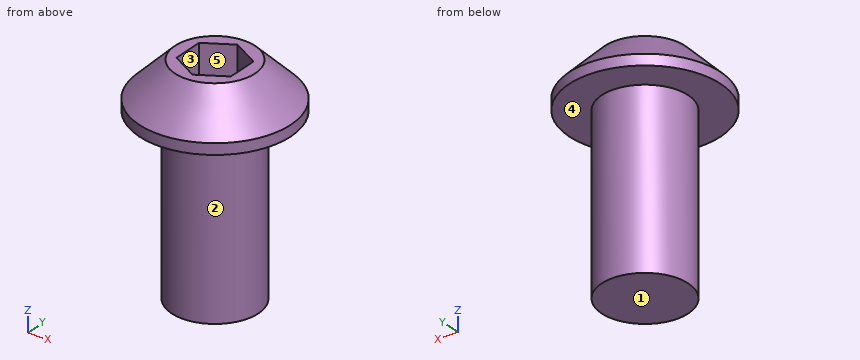
```python
from build123d import *

# Parameters (mm, degrees)
SKETCH1_R           = 7
BASE_EXTRUDE_DEPTH  = 4.3
SKETCH2_R           = 4
BOSS_EXTRUDE1_DEPTH = 16
CUT_EXTRUDE1_DEPTH  = 4.3
CHAMFER1_SIZE       = 3.3


with BuildPart() as part:
    # Sketch1 → Base-Extrude (new body)
    with BuildSketch(Plane.XY):
        Circle(SKETCH1_R)
    extrude(amount=BASE_EXTRUDE_DEPTH)

    # Sketch2 → Boss-Extrude1 (add)
    with BuildSketch(Plane(origin=(0, 0, 0), x_dir=(-1, 0, 0), z_dir=(0, 0, -1))):
        Circle(SKETCH2_R)
    extrude(amount=BOSS_EXTRUDE1_DEPTH)

    # Sketch3 → Cut-Extrude1 (cut)
    with BuildSketch(Plane.XY.offset(4.3)):
        Polygon((0, 2.886751346), (-2.5, 1.443375673), (-2.5, -1.443375673), (0, -2.886751346), (2.5, -1.443375673), (2.5, 1.443375673), align=None)
    extrude(amount=-CUT_EXTRUDE1_DEPTH, mode=Mode.SUBTRACT)

    # Chamfer1
    chamfer1_edges = [part.edges().sort_by_distance(p)[0] for p in [
        (-7, 0, 4.3),
    ]]
    chamfer(chamfer1_edges, length=CHAMFER1_SIZE)


solid = part.part
```
Model file for the job. Use its own axes, mm. Face numbers are marked on the shaded views. A direction names the side the tool comes from. Give positions to 0.01 mm unless a question says otherwise; leave off trailing zeros. Loops run counter-clockwise (first coordinate to the right, second up) from the corner with the lowest first, then second, coordinate; pieces in that order, holes last. Notation, with made-up numbers: (56, -37) - (106, -37) arc R32 ccw to (106, -8) - close; hole circle Ø8 at (39, 53.25). An arc over 180 degrees is marked (long way). One line per item, written item: value. Start each with the question number.
1. Which spindle directions (+Z, -Z, +X, -X, +Y, -Y) get a long thin tool onto all of the face, cutting with end or side? Do the marked faces 4 and 5. Say none if no direction does.
2. Probe L1, parallel to Z at x = 2, y = -1.25; L2, parallel to Y at x = 0, z = -7; L3, parallel to X at y = -2.5, z = 1.25. List the from-to ranges inside material, lowest first. Write a range as from..to.
3. Slice it at B-B (z = -2.5). List the corners of the cut face in (x, y), plus the area to 3 significant figures.
4. Pin check, flat tips, straight feed: pin 1 (3 mm diameter, centred on y = 1, z = -8, fed in from -X); pin 2 (1 mm diameter, centred on y = 5, z = 2, fed in from +X); pin 3 (3 mm diameter, centred on x = -1.5, z = 2, fed in from +Y). Stop position of each tip, or through.
5. Pull direction Y, two halves, no side cores. Call the marked faces 1, 2 and 3: pulls with the +Y half, pulls with the -Y half, needs draft (parallel to the pull), parting line crosses it, or undercut.
6. Slice it at A-A (y = 0). List the corners of the cut face in (x, z), plus the area to 3 significant figures.
Solution:
1. face 4: -Z
1. face 5: +Z
2. L1: z = -16..0
2. L2: y = -4..4
2. L3: x = -6.27..-0.67, 0.67..6.27
3. outline: circle Ø8 at (0, 0)
3. area: 50.3 mm^2
4. pin 1: stops at x = -4
4. pin 2: stops at x = 4.34
4. pin 3: stops at y = 6.99
5. face 1: needs draft
5. face 2: parting line crosses it
5. face 3: undercut
6. outline: (-7, 0) - (-4, 0) - (-4, -16) - (4, -16) - (4, 0) - (7, 0) - (7, 1) - (3.7, 4.3) - (2.5, 4.3) - (2.5, 0) - (-2.5, 0) - (-2.5, 4.3) - (-3.7, 4.3) - (-7, 1) - close
6. area: 156 mm^2
